The model under review builds one solid part; all positions refer to its coordinate system, in mm. Face numbers are marked on the shaded views. A direction names the side the tool comes from. Coordinates: 2 decimals unless noted, no trailing zeros. Write each loop counter-clockwise with the first axis right and the second up, starting at its lowest first coordinate (ties: lowest second). Pieces come first, ordered by that corner, then holes. Notation, with made-up numbers: (-17.75, -37) - (3.25, -37) arc R17 ccw to (3.25, -8) - close; hole circle Ø3 at (-11.75, 49). An arc over 180 degrees is marked (long way). Put each result on its own line as item: value. Start each with the question number.
Item 1: Mouldability with a two-part tool opening along Y and no side actions: class the marked faces 5, 6, 7 and 8 as pulls with the +Y half, pulls with the -Y half, needs draft (parallel to the pull), parting line crosses it, or undercut.
Item 2: To check wall thickness, follow L1, parallel to Y at x = -20, z = 0; L2, parallel to X at y = -3.5, z = -6.25; L3, parallel to Z at x = -25.5, y = -6.5. State the ranges of each line that lie inside material, in increasing order. Write a range as [from, to].
Item 3: For pin 1 (0.6 mm diameter, centred on x = -1, z = 0.5, fed in from -Y); pin 2 (0.6 mm diameter, centred on x = -1.5, z = 1.5, fed in from +Y); pin 3 (12 mm diameter, centred on x = -6, y = 6.5, fed in from -Z); pin 4 (6.5 mm diameter, centred on y = -0.5, z = -1.5, fed in from -X), all flat-tipped, find the tip position at first contact; note any pin that passes through.
Item 4: Consider section A-A on z = 0. Give the boundary of the cut face in (x, y), then the cut area to 3 significant figures.
Item 5: Consider section C-C on y = 9.5. Give the boundary of the cut face in (x, z).
Item 6: Machinability: for the marked faces 1, 2, 3 and 4, which of the approach directions +Z, -Z, +X, -X, +Y, -Y give a long, thin tool a straight path to every point of the face, cutting with its end or side? Answer none if there is none.
Item 7: Consider section B-B on x = -13.5. Give the boundary of the cut face in (y, z), then the cut area to 3 significant figures.
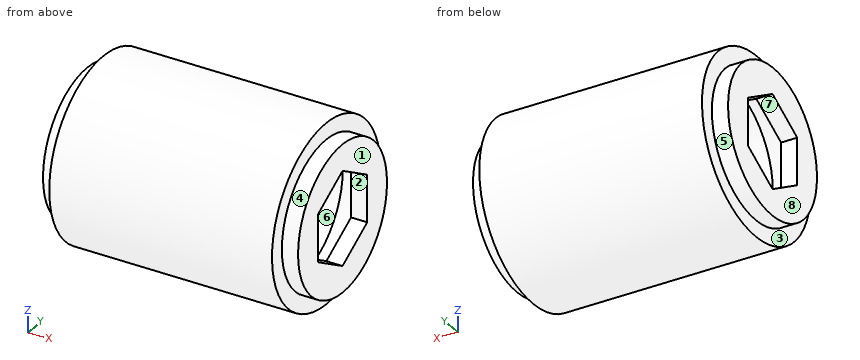
```python
from build123d import *

# Parameters (mm, degrees)
CUT_EXTRUDE1_DEPTH = 36.167763648


with BuildPart() as part:
    # Sketch4 → Revolve2 (revolve)
    with BuildSketch(Plane.XY, mode=Mode.PRIVATE) as revolve2_sk:
        Polygon((-29.54, 11), (-2, 11), (-2, 9), (0, 9), (0, 7), (0, 0), (-2, 0), (-2, 7), (-5.464101615, 9), (-26.075898385, 9), (-29.54, 7), (-29.54, 0), (-31.54, 0), (-31.54, 7), (-31.54, 9), (-29.54, 9), align=None)
    revolve(revolve2_sk.sketch.rotate(Axis((0, 0, 0), (-1, 0, 0)), 90), axis=Axis((0, 0, 0), (-1, 0, 0)))

    # Sketch5 → Cut-Extrude1 (cut, through all)
    with BuildSketch(Plane.ZY.offset(31.54)):
        Polygon((-2.886751346, 5), (-5.773502692, 0), (-2.886751346, -5), (2.886751346, -5), (5.773502692, 0), (2.886751346, 5), align=None)
    extrude(amount=-CUT_EXTRUDE1_DEPTH, mode=Mode.SUBTRACT)


solid = part.part
```
Report:
1. face 5: parting line crosses it
1. face 6: undercut
1. face 7: undercut
1. face 8: needs draft
2. L1: [-11, -9], [9, 11]
2. L2: [-31.54, -29.26], [-2.28, 0]
2. L3: [-8.87, -6.22], [6.22, 8.87]
3. pin 1: y = -9
3. pin 2: y = 8.92
3. pin 3: z = -10.99
3. pin 4: through
4. outline: (-31.54, -9) - (-29.54, -9) - (-29.54, -11) - (-2, -11) - (-2, -9) - (0, -9) - (0, -5) - (-2, -5) - (-2, -7) - (-5.46, -9) - (-26.08, -9) - (-29.54, -7) - (-29.54, -5) - (-31.54, -5) - close; (-31.54, 5) - (-29.54, 5) - (-29.54, 7) - (-26.08, 9) - (-5.46, 9) - (-2, 7) - (-2, 5) - (0, 5) - (0, 9) - (-2, 9) - (-2, 11) - (-29.54, 11) - (-29.54, 9) - (-31.54, 9) - close
4. area: 156 mm²
5. outline: (-29.54, -5.55) - (-2, -5.55) - (-2, 5.55) - (-29.54, 5.55) - close
6. face 1: +Z, -Z, +X, +Y, -Y
6. face 2: +X, -X
6. face 3: -X
6. face 4: +X
7. outline: circle Ø22 at (0, 0); hole circle Ø18 at (0, 0)
7. area: 126 mm²
